from build123d import *

# Parameters (mm, degrees)
SKETCH1_W           = 19.5
SKETCH1_H           = 14.5
BOSS_EXTRUDE1_DEPTH = 10
SKETCH2_R           = 2.5
CUT_EXTRUDE1_DEPTH  = 10
SHELL1_T            = -2
FILLET1_R           = 2
SKETCH3_W           = 15.5
SKETCH3_H           = 1
CUT_EXTRUDE3_DEPTH  = 8
FILLET2_R           = 2
SKETCH4_W           = 5
SKETCH4_H           = 14.507593663
SKETCH4_H_2         = 14.440076449
BOSS_EXTRUDE2_DEPTH = 2
FILLET3_R           = 2
FILLET4_R           = 2
SKETCH5_W           = 5
SKETCH5_H           = 6
CUT_EXTRUDE4_DEPTH  = 22
SKETCH6_W           = 3
SKETCH6_H           = 4.886451311
BOSS_EXTRUDE3_DEPTH = 2
FILLET5_R           = 1


# Some blends are built 0.0001 mm under size
with BuildPart() as part:
    # Sketch1 → Boss-Extrude1 (new body)
    with BuildSketch(Plane(origin=(0, 0, 0), x_dir=(1, 0, 0), z_dir=(0, 1, 0))):
        with Locations((-15.762004242, 10.336365648)):
            Rectangle(SKETCH1_W, SKETCH1_H)
    extrude(amount=BOSS_EXTRUDE1_DEPTH)

    # Sketch2 → Cut-Extrude1 (cut)
    with BuildSketch(Plane(origin=(0, 10, 0), x_dir=(1, 0, 0), z_dir=(0, 1, 0))):
        with Locations((-15.762004242, 4.966482791)):
            Circle(SKETCH2_R)
    extrude(amount=-CUT_EXTRUDE1_DEPTH, mode=Mode.SUBTRACT)

    # Shell1
    shell1_openings = [part.faces().sort_by_distance(p)[0] for p in [
        (-15.762004242, 10, -10.695281365),
    ]]
    offset(amount=SHELL1_T, openings=shell1_openings, kind=Kind.INTERSECTION)

    # Fillet1
    fillet1_edges = [part.edges().sort_by_distance(p)[0] for p in [
        (-17.409778355, 5, -3.086365648),
        (-14.114230128, 5, -3.086365648),
    ]]
    fillet(fillet1_edges, radius=FILLET1_R)

    # Sketch3 → Cut-Extrude3 (cut)
    with BuildSketch(Plane(origin=(0, 10, 0), x_dir=(1, 0, 0), z_dir=(0, 1, 0))):
        with Locations((-15.762004242, 16.086365648)):
            Rectangle(SKETCH3_W, SKETCH3_H)
    extrude(amount=-CUT_EXTRUDE3_DEPTH, mode=Mode.SUBTRACT)

    # Fillet2
    # the kernel refuses this fillet: 2 mm, written as the material it adds along each edge
    with BuildSketch(Plane(origin=(-15.762004242, 2, -4.966482791), x_dir=(0.4658564831234789, 0, 0.8848602924370738), z_dir=(-0.8848602924370738, 0, 0.4658564831234789))) as fillet2_piece_1_section:
        with BuildLine():
            CenterArc((4.5 + FILLET2_R, FILLET2_R), FILLET2_R, 180, 90)
            Line((4.5, FILLET2_R), (4.5, 0))
            Line((4.5, 0), (4.5 + FILLET2_R, 0))
        make_face()
    fillet2_piece_1 = revolve(axis=Axis((-15.762004242, 2, -4.966482791), (0, 1, 0)), revolution_arc=304.468667484, mode=Mode.PRIVATE)
    fillet2_piece_1 = split(fillet2_piece_1, bisect_by=Plane(origin=(-15.762004242, 2.56810824, -5.086365648), z_dir=(0, 0, -1)), keep=Keep.TOP, mode=Mode.PRIVATE)
    add(fillet2_piece_1)
    with BuildSketch(Plane(origin=(-8.012004242, 2, -16.586365648), x_dir=(-1, 0, 0), z_dir=(0, 0, 1)), Plane(origin=(-23.512004242, 2, -5.086365648), x_dir=(1, 0, 0), z_dir=(0, 0, -1))) as fillet2_piece_2:
        with BuildLine():
            CenterArc((FILLET2_R, -FILLET2_R), FILLET2_R, 90, 90)
            Line((0, -FILLET2_R), (0, 0))
            Line((0, 0), (FILLET2_R, 0))
        make_face()
    extrude(amount=11.5)
    with BuildSketch(Plane(origin=(-8.012004242, 2, -16.586365648), x_dir=(0, 1, 0), z_dir=(-1, 0, 0))) as fillet2_piece_3:
        with BuildLine():
            CenterArc((FILLET2_R, -FILLET2_R), FILLET2_R, 90, 90)
            Line((0, -FILLET2_R), (0, 0))
            Line((0, 0), (FILLET2_R, 0))
        make_face()
    extrude(amount=15.5)

    # Sketch4 → Boss-Extrude2 (add)
    with BuildSketch(Plane(origin=(0, 10, 0), x_dir=(1, 0, 0), z_dir=(0, 1, 0))):
        with Locations((-26.012004242, 10.332568817)):
            Rectangle(SKETCH4_W, SKETCH4_H)
        with Locations((-5.512004242, 10.366327424)):
            Rectangle(SKETCH4_W, SKETCH4_H_2)
    extrude(amount=BOSS_EXTRUDE2_DEPTH)

    # Fillet3
    fillet3_edges = [part.edges().sort_by_distance(p)[0] for p in [
        (-8.012004242, 10, -4.116327424),
        (-23.512004242, 10, -4.086365648),
    ]]
    fillet(fillet3_edges, radius=FILLET3_R - 0.0001)  # a hair under: the kernel refuses the full size

    # Fillet4
    fillet4_edges = [part.edges().sort_by_distance(p)[0] for p in [
        (-23.512004242, 10, -17.086365648),
        (-8.012004242, 10, -17.086365648),
    ]]
    fillet(fillet4_edges, radius=FILLET4_R - 0.0001)  # a hair under: the kernel refuses the full size

    # Sketch5 → Cut-Extrude4 (cut)
    with BuildSketch(Plane.ZY.offset(25.512004242)):
        with Locations((-10.415649008, 6.599188408)):
            Rectangle(SKETCH5_W, SKETCH5_H)
    extrude(amount=-CUT_EXTRUDE4_DEPTH, mode=Mode.SUBTRACT)

    # Sketch6 → Boss-Extrude3 (add)
    with BuildSketch(Plane(origin=(0, 3.599188408, 0), x_dir=(1, 0, 0), z_dir=(0, 1, 0))):
        with Locations((-24.971430195, 10.472423353)):
            Rectangle(SKETCH6_W, SKETCH6_H)
        with Locations((-6.552578288, 10.472423353)):
            Rectangle(SKETCH6_W, SKETCH6_H)
    extrude(amount=BOSS_EXTRUDE3_DEPTH)

    # Fillet5
    # the kernel refuses this fillet: 1 mm, written as the material it takes off along each edge
    with BuildSketch(Plane(origin=(-5.052578288, 3.599188408, -15.415649008), x_dir=(0, 1, 0), z_dir=(0, 0, 1))) as fillet5_piece_1_section:
        with BuildLine():
            CenterArc((FILLET5_R, FILLET5_R), FILLET5_R, 180, 90)
            Line((0, FILLET5_R), (0, 0))
            Line((0, 0), (FILLET5_R, 0))
        make_face()
    fillet5_piece_1 = extrude(amount=9.886451311, mode=Mode.PRIVATE)
    fillet5_piece_1 = split(fillet5_piece_1, bisect_by=Plane(origin=(-6.012004242, 3.822567924, -10.472423353), z_dir=(1, 0, 0)), keep=Keep.TOP, mode=Mode.PRIVATE)
    add(fillet5_piece_1, mode=Mode.SUBTRACT)
    with BuildSketch(Plane(origin=(-5.052578288, 5.599188408, -12.915649008), x_dir=(-1, 0, 0), z_dir=(0, 0, 1))) as fillet5_piece_2:
        with BuildLine():
            CenterArc((FILLET5_R, FILLET5_R), FILLET5_R, 180, 90)
            Line((0, FILLET5_R), (0, 0))
            Line((0, 0), (FILLET5_R, 0))
        make_face()
    extrude(amount=4.886451311, mode=Mode.SUBTRACT)
    with BuildSketch(Plane(origin=(-26.471430195, 3.599188408, -15.415649008), x_dir=(1, 0, 0), z_dir=(0, 0, 1))) as fillet5_piece_3_section:
        with BuildLine():
            CenterArc((FILLET5_R, FILLET5_R), FILLET5_R, 180, 90)
            Line((0, FILLET5_R), (0, 0))
            Line((0, 0), (FILLET5_R, 0))
        make_face()
    fillet5_piece_3 = extrude(amount=9.886451311, mode=Mode.PRIVATE)
    fillet5_piece_3 = split(fillet5_piece_3, bisect_by=Plane(origin=(-25.512004242, 3.822567924, -10.472423353), z_dir=(-1, 0, 0)), keep=Keep.TOP, mode=Mode.PRIVATE)
    add(fillet5_piece_3, mode=Mode.SUBTRACT)
    with BuildSketch(Plane(origin=(-26.471430195, 5.599188408, -12.915649008), x_dir=(1, 0, 0), z_dir=(0, 0, 1))) as fillet5_piece_4:
        with BuildLine():
            CenterArc((FILLET5_R, -FILLET5_R), FILLET5_R, 90, 90)
            Line((0, -FILLET5_R), (0, 0))
            Line((0, 0), (FILLET5_R, 0))
        make_face()
    extrude(amount=4.886451311, mode=Mode.SUBTRACT)


solid = part.part
Source: CAD feature listing. Evaluate the final solid. Frame: model axes, mm. A direction names the side the tool comes from. Round coordinates to 2 decimals unless told otherwise and drop trailing zeros. Order: outer loops, then holes, each group sorted by start corner. A loop starts at its lowest first (then second) coordinate and runs counter-clockwise, first axis right, second up. Notation, with made-up numbers: (59, 15) - (106, 15) arc R20 cw to (106, 23) - close; hole circle Ø7 at (58.25, -36). An arc over 180 degrees is marked (long way). Use a Markdown table: item, result. Add a question column.
1. Section query C-C (x = -22.75). Return the cut outline in (y, z), then the cut area to 3 significant figures.
2. Section query D-D (z = -15.25). Return the cut outline in (x, y), then the cut area to 3 significant figures.
3. Line query: probe 1 along Z at (x, y) = (-7.5, 5.75); probe 2 along X at (y, z) = (7.25, -14.25); probe 3 along X at (y, z) = (10.5, -15.75). Output: solid intervals per line, ascending.
4. Set-up query: faces 4 (the flat face through (-25, 9.599, -10)), 5 (the flat face through (-3.012, 11, -10)), 6 (the flat face through (-16, 10, -17)), 7 (the cylindrical face through (-15.654, 2.601, -16.016)), 8 (the flat face through (-6, 11, -3.146)). Return all of +Z, -Z, +X, -X, +Y, -Y with unobstructed straight access to the full face (end or side cutting, diameter ignored); none if empty.
5. Section query B-B (y = 6). Return the cut outline in (x, z), then the cut area to 3 significant figures.
6. Section query A-A (z = -12.5). Return the cut outline in (x, y).
7. Mould query, pull axis Z, two halves, no side actions, for faces 1 (the flat face through (-7, 7, -7.916)), 2 (the cylindrical face through (-12.6, 5.1, -3.6)), 3 (the cylindrical face through (-8.582, 10.601, -17.093)). Classes: +Z half, -Z half, draft (parallel to the pull), parting line (faces both ways), or undercut.
8. First-contact query: pin 1 (5 mm diameter, centred on x = -14.5, y = 3, fed in from +Z); pin 2 (4 mm diameter, centred on x = -15.5, y = 7.5, fed in from +Z); pin 3 (4 mm diameter, centred on x = -19.5, y = 10, fed in from +Z); pin 4 (1.5 mm diameter, centred on x = -16, z = -6, fed in from -Y) (1 decimal). Flat tips, straight axial feed; report the tip coordinate or a pass-through.
Derived:
| question | item | result |
|---|---|---|
| 1 | outline | (0, -17.59) - (10.43, -17.59) - (10.43, -16.59) - (4, -16.59) arc R2 cw to (2.43, -15.82) - (2.43, -5.09) - (10.43, -5.09) - (10.43, -3.09) - (0, -3.09) - close |
| 1 | area | 59.6 mm2 |
| 2 | outline | (-28.51, 10) - (-25.51, 10) - (-25.51, 0) - (-6.01, 0) - (-6.01, 10) - (-3.01, 10) - (-3.01, 12) - (-8.01, 12) - (-8.01, 4) arc R2 cw to (-9.35, 2.11) - (-22.18, 2.11) arc R2 cw to (-23.51, 4) - (-23.51, 12) - (-28.51, 12) - close |
| 2 | area | 94.1 mm2 |
| 3 | probe 1 | -17.59 to -12.92, -7.92 to -3.09 |
| 3 | probe 2 | -25.51 to -23.51, -8.01 to -6.01 |
| 3 | probe 3 | -28.51 to -23.51, -8.01 to -3.01 |
| 4 | face 4 | +X, -X |
| 4 | face 5 | +Z, -Z, +X, +Y, -Y |
| 4 | face 6 | +Z, -Z, +Y |
| 4 | face 7 | +Y |
| 4 | face 8 | +Z, +X, +Y |
| 5 | outline | (-25.51, -17.59) - (-6.01, -17.59) - (-6.01, -12.92) - (-8.01, -12.92) - (-8.01, -16.59) - (-23.51, -16.59) - (-23.51, -12.92) - (-25.51, -12.92) - close; (-25.51, -7.92) - (-23.51, -7.92) - (-23.51, -5.09) - (-20.26, -5.09) arc R4.5 ccw to (-19.16, -7.92) - (-12.36, -7.92) arc R4.5 ccw to (-11.26, -5.09) - (-8.01, -5.09) - (-8.01, -7.92) - (-6.01, -7.92) - (-6.01, -3.09) - (-11.26, -3.09) arc R2 ccw to (-13.26, -5.03) arc R2.5 cw to (-18.26, -5.03) arc R2 ccw to (-20.26, -3.09) - (-25.51, -3.09) - close |
| 5 | area | 87.0 mm2 |
| 6 | outline | (-28.51, 10) - (-25.51, 10) - (-25.51, 9.6) - (-23.51, 9.6) - (-23.51, 12) - (-28.51, 12) - close; (-25.51, 0) - (-6.01, 0) - (-6.01, 3.6) arc R1 ccw to (-6.05, 5.6) - (-8.05, 5.6) - (-8.05, 3.6) arc R2 cw to (-10.01, 2) - (-21.51, 2) arc R2 cw to (-23.47, 3.6) - (-23.47, 5.6) - (-25.47, 5.6) arc R1 ccw to (-25.51, 3.6) - close; (-8.01, 9.6) - (-6.01, 9.6) - (-6.01, 10) - (-3.01, 10) - (-3.01, 12) - (-8.01, 12) - close |
| 7 | face 1 | undercut |
| 7 | face 2 | +Z half |
| 7 | face 3 | draft |
| 8 | pin 1 | z = -3.23 |
| 8 | pin 2 | z = -6.03 |
| 8 | pin 3 | z = -3.09 |
| 8 | pin 4 | through |
